Build history of the part. All positions in model axes, mm. A direction names the side the tool comes from. Give positions to 0.01 mm unless a question says otherwise; leave off trailing zeros. Order: outer loops, then holes, each group sorted by start corner. A loop starts at its lowest first (then second) coordinate and runs counter-clockwise, first axis right, second up. Notation, with made-up numbers: (-21, 73.5) - (32, 73.5) arc R30 cw to (32, 110.5) - close; hole circle Ø5 at (31.25, 82). An arc over 180 degrees is marked (long way). Use a Markdown table: item, result.
from build123d import *

# Parameters (mm, degrees)
SKETCH1_W           = 19
SKETCH1_H           = 22.5
BOSS_EXTRUDE1_DEPTH = 37
BOSS_EXTRUDE2_DEPTH = 11
FILLET1_R           = 5
SKETCH3_R           = 1.5
CUT_EXTRUDE1_DEPTH  = 20
SKETCH4_W           = 2.5
SKETCH4_H           = 5
BOSS_EXTRUDE3_DEPTH = 5
FILLET2_R           = 0.5
SKETCH5_R           = 1.5
CUT_EXTRUDE2_DEPTH  = 5
SKETCH6_R           = 2.8
CUT_EXTRUDE3_DEPTH  = 20
CUT_EXTRUDE4_DEPTH  = 11
SKETCH8_R           = 3
CUT_EXTRUDE5_DEPTH  = 2


with BuildPart() as part:
    # Sketch1 → Boss-Extrude1 (new body)
    with BuildSketch(Plane.XY):
        Rectangle(SKETCH1_W, SKETCH1_H)
    extrude(amount=BOSS_EXTRUDE1_DEPTH)

    # Sketch2 → Boss-Extrude2 (add)
    with BuildSketch(Plane(origin=(0, 0, 0), x_dir=(-1, 0, 0), z_dir=(0, 0, -1))):
        with BuildLine():
            Line((9.5, 6.025985397), (9.5, -6.025985397))
            ThreePointArc((9.5, -6.025985397), (0, -11.25), (-9.5, -6.025985397))
            Line((-9.5, -6.025985397), (-9.5, 6.025985397))
            ThreePointArc((-9.5, 6.025985397), (0, 11.25), (9.5, 6.025985397))
        make_face()
    extrude(amount=BOSS_EXTRUDE2_DEPTH)

    # Fillet1
    fillet1_edges = [part.edges().sort_by_distance(p)[0] for p in [
        (0, 11.25, 37),
        (0, -11.25, 37),
    ]]
    fillet(fillet1_edges, radius=FILLET1_R)

    # Sketch3 → Cut-Extrude1 (cut, through all)
    with BuildSketch(Plane(origin=(9.5, 0, 0), x_dir=(0, 0, -1), z_dir=(1, 0, 0))):
        with Locations((-5, 8.75)):
            Circle(SKETCH3_R)
        with Locations((-5, -8.75)):
            Circle(SKETCH3_R)
    extrude(amount=-CUT_EXTRUDE1_DEPTH, mode=Mode.SUBTRACT)

    # Sketch4 → Boss-Extrude3 (add)
    with BuildSketch(Plane.XY.offset(37)):
        Rectangle(SKETCH4_W, SKETCH4_H)
    extrude(amount=BOSS_EXTRUDE3_DEPTH)

    # Fillet2
    fillet2_edges = [part.edges().sort_by_distance(p)[0] for p in [
        (-9.5, 0, 37),
        (9.5, 0, 37),
        (9.5, 11.25, 16),
        (9.5, -11.25, 16),
        (9.5, 9.785533906, 35.535533906),
        (9.5, -9.785533906, 35.535533906),
        (-9.5, -11.25, 16),
        (-9.5, 11.25, 16),
        (-9.5, 9.785533906, 35.535533906),
        (-9.5, -9.785533906, 35.535533906),
        (0, -2.5, 42),
        (0, 2.5, 42),
    ]]
    fillet(fillet2_edges, radius=FILLET2_R)

    # Sketch5 → Cut-Extrude2 (cut)
    with BuildSketch(Plane(origin=(1.25, 0, 0), x_dir=(0, 0, -1), z_dir=(1, 0, 0))):
        with Locations((-39.5, 0)):
            Circle(SKETCH5_R)
    extrude(amount=-CUT_EXTRUDE2_DEPTH, mode=Mode.SUBTRACT)

    # Sketch6 → Cut-Extrude3 (cut, through all)
    with BuildSketch(Plane(origin=(9.5, 0, 0), x_dir=(0, 0, -1), z_dir=(1, 0, 0))):
        with Locations((-25.5, 0)):
            Circle(SKETCH6_R)
    extrude(amount=-CUT_EXTRUDE3_DEPTH, mode=Mode.SUBTRACT)

    # Sketch7 → Cut-Extrude4 (cut)
    with BuildSketch(Plane(origin=(0, 0, -11), x_dir=(-1, 0, 0), z_dir=(0, 0, -1))):
        with BuildLine():
            Line((-8.3, 5.666789214), (-8.3, -5.666789214))
            ThreePointArc((-8.3, -5.666789214), (0, -10.05), (8.3, -5.666789214))
            Line((8.3, -5.666789214), (8.3, 5.666789214))
            ThreePointArc((8.3, 5.666789214), (0, 10.05), (-8.3, 5.666789214))
        make_face()
    extrude(amount=-CUT_EXTRUDE4_DEPTH, mode=Mode.SUBTRACT)

    # Sketch8 → Cut-Extrude5 (cut)
    with BuildSketch(Plane(origin=(0, 0, 0), x_dir=(-1, 0, 0), z_dir=(0, 0, -1))):
        Circle(SKETCH8_R)
    extrude(amount=-CUT_EXTRUDE5_DEPTH, mode=Mode.SUBTRACT)


solid = part.part
1) Tool access for faces 1 (the flat face through (1.25, -1, 41)), 2 (the flat face through (-7, 10, 0)), 3 (the cylindrical face through (0.14, -10.05, -5.58)), 4 (the cylindrical face through (0.16, 11.25, -5.42)), 5 (the flat face through (-7, -10, 0)): list every direction of +Z, -Z, +X, -X, +Y, -Y with a clear straight run to the whole face (end or side of a thin tool).
Computed:
| item | result |
|---|---|
| face 1 | +Z, +X, +Y, -Y |
| face 2 | -Z, -X, +Y |
| face 3 | -Z |
| face 4 | -Z, +Y |
| face 5 | -Z, -X, -Y |
2) Wall check: line 1 (Y direction, x = 0, z = 1.45); line 2 (Z direction, x = 7.5, y = 0.25); line 3 (Y direction, x = 3.75, z = 4.5). Give the ranges that are in metal, low to high. Write a range as from..to.
Computed:
| item | result |
|---|---|
| line 1 | y = -11.25..-3, 3..11.25 |
| line 2 | z = 0..22.71, 28.29..37 |
| line 3 | y = -11.25..-10.16, -7.34..7.34, 10.16..11.25 |
3) Pin check, flat tips, straight feed: P1, Ø8.5, axis at x = -0.5, y = 4, coming from the -Z side; P2, Ø3.5, axis at y = 0, z = 39.5, coming from the -X side; P3, Ø5.5, axis at x = 0, y = 0, coming from the -Z side. Stop position of each tip, or through.
Computed:
| item | result |
|---|---|
| P1 | stops at z = 0 |
| P2 | stops at x = -1.25 |
| P3 | stops at z = 2 |
4) Slice it at B-B (y = 0). Write the cut outline in (x, z), and give its area (3 significant figures).
Computed:
| item | result |
|---|---|
| outline | (-9.5, -11) - (-8.3, -11) - (-8.3, 0) - (-3, 0) - (-3, 2) - (3, 2) - (3, 0) - (8.3, 0) - (8.3, -11) - (9.5, -11) - (9.5, 22.7) - (-9.5, 22.7) - close; (-9.5, 28.3) - (9.5, 28.3) - (9.5, 36.5) arc R0.5 ccw to (9, 37) - (1.25, 37) - (1.25, 38) - (-1.25, 38) - (-1.25, 37) - (-9, 37) arc R0.5 ccw to (-9.5, 36.5) - close; (-1.25, 41) - (1.25, 41) - (1.25, 42) - (-1.25, 42) - close |
| area | 616 mm² |
5) Slice it at A-A (z = 39.5). Write the cut outline in (x, y), and give its area (3 significant figures).
Computed:
| item | result |
|---|---|
| outline | (-1.25, -2.5) - (1.25, -2.5) - (1.25, -1.5) - (-1.25, -1.5) - close; (-1.25, 1.5) - (1.25, 1.5) - (1.25, 2.5) - (-1.25, 2.5) - close |
| area | 5.00 mm² |
6) Slice it at C-C (x = 5.25). Write the cut outline in (y, z).
Computed:
| item | result |
|---|---|
| outline | (-11.25, 0) - (-9.95, 0) - (-9.95, -11) - (-8.57, -11) - (-8.57, 0) - (8.57, 0) - (8.57, -11) - (9.95, -11) - (9.95, 0) - (11.25, 0) - (11.25, 32) arc R5 ccw to (6.25, 37) - (-6.25, 37) arc R5 ccw to (-11.25, 32) - close; hole circle Ø3 at (-8.75, 5); hole circle Ø5.6 at (0, 25.5); hole circle Ø3 at (8.75, 5) |
7) Slice it at D-D (z = -5.5). Write the cut outline in (x, y).
Computed:
| item | result |
|---|---|
| outline | (-9.5, -6.03) arc R11.25 ccw to (9.5, -6.03) - (9.5, 6.03) arc R11.25 ccw to (-9.5, 6.03) - close; hole (-8.3, -5.67) arc R10.05 ccw to (8.3, -5.67) - (8.3, 5.67) arc R10.05 ccw to (-8.3, 5.67) - close |
8) Two-plate mould, pull along Y, no slides. Class faces 6 (the cylindrical face through (0.1, 0.1, 28.3)), 7 (the flat face through (-8.5, 0.9, -11)), 8 (the flat face through (0, 2.5, 39)): +Y half, -Y half, draft (parallel to the pull), parting line (faces both ways), or undercut.
Computed:
| item | result |
|---|---|
| face 6 | undercut |
| face 7 | draft |
| face 8 | +Y half |
